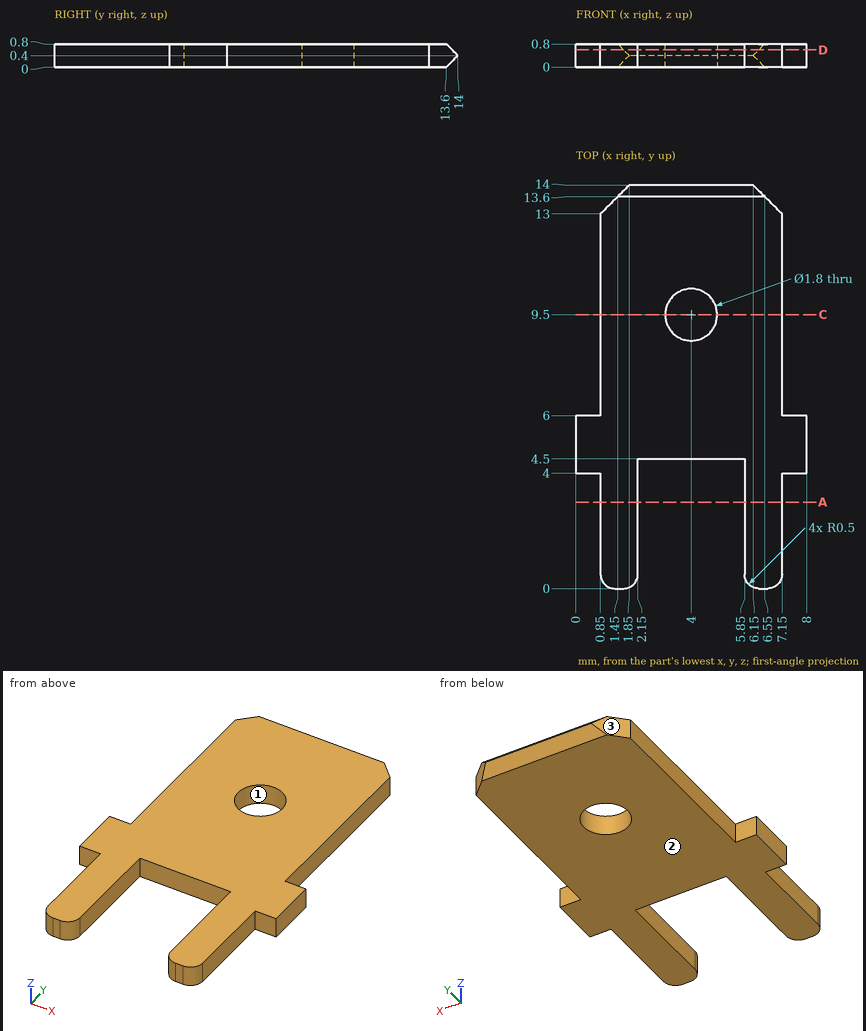
For this review, use the dimensioned drawing (mm, ordinates from the lowest corner) and the shaded views. Coordinates: 2 decimals unless noted, no trailing zeros. Order: outer loops, then holes, each group sorted by start corner. A loop starts at its lowest first (then second) coordinate and runs counter-clockwise, first axis right, second up. Notation, with made-up numbers: (2, 67) - (33, 67) arc R26 cw to (33, 98) - close; hole circle Ø2 at (50.25, -18.75). An arc over 180 degrees is marked (long way). Answer in a Markdown table with one row per item.
(1) Consider section D-D on z = 0.6. State the section outline as (x, y) points.
Checked values:
| item | result |
|---|---|
| outline | (0, 4) - (0.85, 4) - (0.85, 0.5) arc R0.5 ccw to (1.35, 0) - (1.65, 0) arc R0.5 ccw to (2.15, 0.5) - (2.15, 4.5) - (5.85, 4.5) - (5.85, 0.5) arc R0.5 ccw to (6.35, 0) - (6.65, 0) arc R0.5 ccw to (7.15, 0.5) - (7.15, 4) - (8, 4) - (8, 6) - (7.15, 6) - (7.15, 13) - (6.35, 13.8) - (1.65, 13.8) - (0.85, 13) - (0.85, 6) - (0, 6) - close; hole circle Ø1.8 at (4, 9.5) |
(2) Clearance check with flat-ended pins moving along their axes: pin 1 (2 mm diameter, centred on x = 2.5, y = 3, fed in from +Z); pin 2 (1.4 mm diameter, centred on x = 4, y = 9.5, fed in from -Z). State where each tip first meets the part, or that it passes through.
Checked values:
| item | result |
|---|---|
| pin 1 | z = 0.8 |
| pin 2 | through |
(3) Consider section A-A on y = 3. State the section outline as (x, z) points, plus the area to 3 significant figures.
Checked values:
| item | result |
|---|---|
| outline | (0.85, 0) - (2.15, 0) - (2.15, 0.8) - (0.85, 0.8) - close; (5.85, 0) - (7.15, 0) - (7.15, 0.8) - (5.85, 0.8) - close |
| area | 2.08 mm^2 |
(4) The part is to be moulded in two halves that separate along X. For the marked faces 1, 2 and 3, say which applies: released by +X, released by -X, zero draft, split by the parting line, or undercut.
Checked values:
| item | result |
|---|---|
| face 1 | undercut |
| face 2 | zero draft |
| face 3 | released by -X |
(5) Wall thickness on line 1 along X through (y, z) = (3, 0.5); line 2 along X through (y, z) = (11.25, 0.5); line 3 along Y through (x, z) = (3.75, 0.1) (1 decimal): over which ranges is each line inside the solid? List them lowest first. Write a range as from..to.
Checked values:
| item | result |
|---|---|
| line 1 | 0.85..2.15, 5.85..7.15 |
| line 2 | 0.85..7.15 |
| line 3 | 4.5..8.6, 10.4..13.7 |
(6) Consider section C-C on y = 9.5. State the section outline as (x, z) points, plus the area to 3 significant figures.
Checked values:
| item | result |
|---|---|
| outline | (0.85, 0) - (3.1, 0) - (3.1, 0.8) - (0.85, 0.8) - close; (4.9, 0) - (7.15, 0) - (7.15, 0.8) - (4.9, 0.8) - close |
| area | 3.60 mm^2 |
